```python
from build123d import *

# Parameters (mm, degrees)
F0_R      = 50
F1_DEPTH  = 40
F2_R      = 10
F3_DEPTH  = 80.001
F4_R      = 37.5
F5_DEPTH  = 10
F6_R      = 22.5
F7_DEPTH  = 20
F8_R      = 37.5
F9_DEPTH  = 10
F10_R     = 22.5
F11_DEPTH = 20


with BuildPart() as f1:
    # F0 (on Front) → F1 (new body, symmetric)
    with BuildSketch(Plane.XZ):
        Circle(F0_R)
    extrude(amount=F1_DEPTH, both=True)

    # F2 (on face) → F3 (cut, through all)
    with BuildSketch(Plane.XZ.offset(40)):
        Circle(F2_R)
    extrude(amount=-F3_DEPTH, mode=Mode.SUBTRACT)

    # F4 (on face) → F5 (cut)
    with BuildSketch(Plane(origin=(0, 40, 0), x_dir=(-1, 0, 0), z_dir=(0, 1, 0))):
        Circle(F4_R)
    extrude(amount=-F5_DEPTH, mode=Mode.SUBTRACT)

    # F6 (on face) → F7 (cut)
    with BuildSketch(Plane(origin=(0, 30, 0), x_dir=(-1, 0, 0), z_dir=(0, 1, 0))):
        Circle(F6_R)
    extrude(amount=-F7_DEPTH, mode=Mode.SUBTRACT)

    # F8 (on face) → F9 (cut)
    with BuildSketch(Plane.XZ.offset(40)):
        Circle(F8_R)
    extrude(amount=-F9_DEPTH, mode=Mode.SUBTRACT)

    # F10 (on face) → F11 (cut)
    with BuildSketch(Plane.XZ.offset(30)):
        Circle(F10_R)
    extrude(amount=-F11_DEPTH, mode=Mode.SUBTRACT)


solid = f1.part
```
Here's how the part is built. I have some questions about the finished solid (model axes, mm). A direction names the side the tool comes from. Give positions to 0.01 mm unless a question says otherwise; leave off trailing zeros. Loops run counter-clockwise (first coordinate to the right, second up) from the corner with the lowest first, then second, coordinate; pieces in that order, holes last. Notation, with made-up numbers: (62.25, -2.5) -> (118.25, -2.5) arc R15 cw to (118.25, 16.5) -> close; hole circle Ø5 at (66, 67.5). An arc over 180 degrees is marked (long way). Use one line per item in the form item = value. Start each with the question number.
1) Imagine slicing it at B-B (x = -8). Please give me the cut outline in (y, z), then the cut area to 3 significant figures.
2) Which directions (+Z, -Z, +X, -X, +Y, -Y) give clear straight access to the entire face, cutting with the end or side of a thin tool? Please do faces 1 (the face through (10.382, -20.14, -19.961)), 2 (the face through (4.88, 35.07, 37.18)), 3 (the face through (7, -40, 37)).
3) Please list where these lines run through material, in increasing order: line 1 along Z through (x, y) = (0, 25); line 2 along Z through (x, y) = (0, -37.5); line 3 along Y through (x, z) = (21, -11).
4) Thinking about a two-plate mould opening in X: for faces 4 (the face through (-16.1, 30, -16.1)), 5 (the face through (7, 40, 37)), 6 (the face through (47.69, -0.56, 15.02)), which applies, +X half, -X half, draft (parallel to the pull), parting line (faces both ways), or undercut?
5) Imagine slicing it at A-A (z = 0). Please give me the cut outline in (x, y), then the cut area to 3 significant figures.
6) Imagine slicing it at D-D (z = -24.5). Please give me the cut outline in (x, y).
7) Imagine slicing it at C-C (y = 3). Please give me the cut outline in (x, z), then the cut area to 3 significant figures.
8) For P1, Ø1, axis at y = 20.5, z = 19, coming from the +X side; P2, Ø12, axis at y = -17, z = 20.5, coming from the +X side; P3, Ø4, axis at y = -18, z = 32.5, coming from the -X side; P4, Ø12, axis at x = 0, z = 0, coming from the +Y side, each with a flat end and sliding along its axis, tell me the tip position at first contact or that it passes through.
Check values:
q1.outline = (-40, -49.36) -> (40, -49.36) -> (40, -36.64) -> (30, -36.64) -> (30, -21.03) -> (10, -21.03) -> (10, -6) -> (-10, -6) -> (-10, -21.03) -> (-30, -21.03) -> (-30, -36.64) -> (-40, -36.64) -> close; (-40, 36.64) -> (-30, 36.64) -> (-30, 21.03) -> (-10, 21.03) -> (-10, 6) -> (10, 6) -> (10, 21.03) -> (30, 21.03) -> (30, 36.64) -> (40, 36.64) -> (40, 49.36) -> (-40, 49.36) -> close
q1.area = 4,510 mm^2
q2.face_1 = -Y
q2.face_2 = +Y
q2.face_3 = +Z, -Z, +X, -X, -Y
q3.line_1 = -50 to -22.5, 22.5 to 50
q3.line_2 = -50 to -37.5, 37.5 to 50
q3.line_3 = -30 to 30
q4.face_4 = undercut
q4.face_5 = draft
q4.face_6 = parting line
q5.outline = (-50, -40) -> (-37.5, -40) -> (-37.5, -30) -> (-22.5, -30) -> (-22.5, -10) -> (-10, -10) -> (-10, 10) -> (-22.5, 10) -> (-22.5, 30) -> (-37.5, 30) -> (-37.5, 40) -> (-50, 40) -> close; (10, -10) -> (22.5, -10) -> (22.5, -30) -> (37.5, -30) -> (37.5, -40) -> (50, -40) -> (50, 40) -> (37.5, 40) -> (37.5, 30) -> (22.5, 30) -> (22.5, 10) -> (10, 10) -> close
q5.area = 4,300 mm^2
q6.outline = (-43.59, -40) -> (-28.39, -40) -> (-28.39, -30) -> (28.39, -30) -> (28.39, -40) -> (43.59, -40) -> (43.59, 40) -> (28.39, 40) -> (28.39, 30) -> (-28.39, 30) -> (-28.39, 40) -> (-43.59, 40) -> close
q7.outline = circle Ø100 at (0, 0); hole circle Ø20 at (0, 0)
q7.area = 7,540 mm^2
q8.P1 = 46.45
q8.P2 = 47.85
q8.P3 = -39.62
q8.P4 = through
